The model under review builds one solid part; all positions refer to its coordinate system, in mm. Face numbers are marked on the shaded views. Give positions to 0.01 mm unless a question says otherwise; leave off trailing zeros. Loops run counter-clockwise (first coordinate to the right, second up) from the corner with the lowest first, then second, coordinate; pieces in that order, holes last. Notation, with made-up numbers: M 50.5,-1.75 L 92.5,-1.75 A13 ccw 92.5,20.25 Z; hole C 2,56 d10. An arc over 180 degrees is marked long. Put each result on its own line as item: value. Start each with the question number.
Autodesk Inventor part; units mm, degrees
ref_plane "YZ Plane" through (0, 0, 0) normal (1, 0, 0) x (0, 1, 0)
ref_plane "XZ Plane" through (0, 0, 0) normal (0, 1, 0) x (-1, 0, 0)
ref_plane "XY Plane" through (0, 0, 0) normal (0, 0, 1) x (1, 0, 0)
sketch "Sketch1" plane through (0, 0, 0) normal (0, 0, 1) x (1, 0, 0)
  circle A0 centre (0, 0) radius 2.5
  line L0 (-1.3162, -2.1255) -> (1.3162, -2.1255)
  circle A1 centre (0, 0) radius 3.175
  dimension "d0" = 5
  dimension "d1" = 6.35
extrude "Extrusion1" add sketch "Sketch1" along normal blind 6.35 contours L0 A0 | A1 picked at (-0.2721, -2.2046)
sketch "Sketch2" plane through (0, 0, 6.35) normal (0, 0, 1) x (1, 0, 0)
  circle A0 centre (0, 0) radius 9.525
  circle A1 centre (0, 0) radius 10.8857
  dimension "d4" = 19.05
  dimension "d5" = 21.7714
extrude "Extrusion2" add sketch "Sketch2" along normal blind 6.35
sketch "Sketch4" plane through (0, 0, 12.7) normal (0, 0, 1) x (1, 0, 0)
  circle A0 centre (0, 0) radius 10.8857
  circle A1 centre (0, 0) radius 9.525
extrude "Extrusion4" add sketch "Sketch4" along normal blind 1.5875 contours A1
sketch "Sketch5" plane through (0, 0, 12.7) normal (0, 0, 1) x (1, 0, 0)
  circle A0 centre (0, 0) radius 10.8857
  circle A1 centre (0, 0) radius 9.525
extrude "Extrusion5" cut sketch "Sketch5" against normal blind 9.525
sketch "Sketch6" plane through (0, 0, 12.7) normal (0, 0, -1) x (-1, 0, 0)
  circle A0 centre (0, 0) radius 9.525
extrude "Extrusion6" add sketch "Sketch6" along normal blind 6.477
fillet "Fillet2" radius 11.1125 1 edges at (-3.175, 0, 6.223)
sketch "Sketch7" plane through (0, 0, 14.2875) normal (0, 0, 1) x (1, 0, 0)
  circle A0 centre (0, 0) radius 9.525
  circle A1 centre (0, 0) radius 4.7625
  dimension "d18" = 9.525
extrude "Extrusion7" cut sketch "Sketch7" against normal blind 15.748
properties part number "Shaft Adapter"
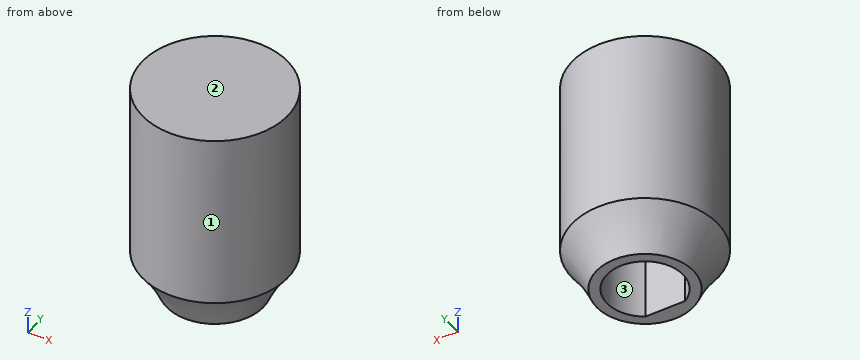
Item 1: Consider section A-A, the plane x = 0. Write out the cut boundary in (y, z) (1 decimal), plus the area to 3 significant figures.
Item 2: Consider section B-B, the plane y = 0. Write out the cut boundary in (x, z) (1 decimal), plus the area to 3 significant figures.
Item 3: Consider section D-D, the plane z = 2.25. Write out the cut boundary in (x, y), plus the area to 3 significant figures.
Item 4: To check wall thickness, follow L1, parallel to Y at x = 0, z = 4.75; L2, parallel to X at y = 0, z = 2; L3, parallel to Y at x = 0, z = 1.5. State the ranges of each line that lie inside material, in increasing order. Write a range as [from, to].
Item 5: Draft analysis for pull direction Y (two halves, no side actions). For the marked faces 1, 2 and 3, state which applies: +Y half, -Y half, draft (parallel to the pull), parting line (faces both ways), or undercut.
Item 6: Consider section C-C, the plane z = 10.75. Write out the cut boundary in (x, y) (1 decimal), plus the area to 3 significant figures.
Report:
1. outline: M -4.8,2.7 A11.1 cw -3.2,0 L -2.1,0 L -2.1,6.2 L 2.5,6.2 L 2.5,0 L 3.2,0 A11.1 cw 4.8,2.7 L 4.8,14.3 L -4.8,14.3 Z
1. area: 102 mm²
2. outline: M -4.8,2.7 A11.1 cw -3.2,0 L -2.5,0 L -2.5,6.2 L 2.5,6.2 L 2.5,0 L 3.2,0 A11.1 cw 4.8,2.7 L 4.8,14.3 L -4.8,14.3 Z
2. area: 100 mm²
3. outline: C 0,0 d8.81; hole M -1.32,-2.13 L 1.32,-2.13 A2.5 ccw long Z
3. area: 41.9 mm²
4. L1: [-4.76, -2.13], [2.5, 4.76]
4. L2: [-4.23, -2.5], [2.5, 4.23]
4. L3: [-3.92, -2.13], [2.5, 3.92]
5. face 1: parting line
5. face 2: draft
5. face 3: undercut
6. outline: C 0,0 d9.5
6. area: 71.3 mm²
